```python
from build123d import *

# Parameters (mm, degrees)
SKETCH2_W           = 20
SKETCH2_H           = 20
SKETCH2_R           = 2.5
BOSS_EXTRUDE1_DEPTH = 250
SKETCH3_R           = 2.5
CUT_EXTRUDE1_DEPTH  = 251.99800796
SKETCH4_R           = 2.5
CUT_EXTRUDE2_DEPTH  = 251.99800796


with BuildPart() as part:
    # Sketch2 → Boss-Extrude1 (new body)
    with BuildSketch(Plane(origin=(0, 0, 0), x_dir=(1, 0, 0), z_dir=(0, 1, 0))):
        Rectangle(SKETCH2_W, SKETCH2_H)
        with Locations(Location((0, 0, 0), (0, 0, 270))):
            Circle(SKETCH2_R, mode=Mode.SUBTRACT)
    extrude(amount=BOSS_EXTRUDE1_DEPTH)

    # Sketch3 → Cut-Extrude1 (cut, through all)
    with BuildSketch(Plane.XY.offset(10)):
        with Locations((0, 5)):
            Circle(SKETCH3_R)
    extrude(amount=-CUT_EXTRUDE1_DEPTH, mode=Mode.SUBTRACT)

    # Sketch4 → Cut-Extrude2 (cut, through all)
    with BuildSketch(Plane.XY.offset(10)):
        with Locations((0, 75)):
            Circle(SKETCH4_R)
        with Locations((0, 85)):
            Circle(SKETCH4_R)
        with Locations((0, 150)):
            Circle(SKETCH4_R)
        with Locations((0, 160)):
            Circle(SKETCH4_R)
    extrude(amount=-CUT_EXTRUDE2_DEPTH, mode=Mode.SUBTRACT)


solid = part.part
```
Could you check a few things on this model? Use its own coordinates, in mm. Give positions to 0.01 mm unless a question says otherwise; leave off trailing zeros. Loops run counter-clockwise (first coordinate to the right, second up) from the corner with the lowest first, then second, coordinate; pieces in that order, holes last. Notation, with made-up numbers: (-2, -5.75) - (56, -5.75) arc R29 cw to (56, 14.25) - close; hole circle Ø1 at (-7.75, 74.25). An arc over 180 degrees is marked (long way). Use one line per item in the form item = value.
1. I'm going to push a flat-ended pin straight in: pin 1 Ø8 at (x, z) = (0, 0) entering from +Y. Where does the tip first touch, or does it pass through?
Response values:
pin_1 = 250
2. Thinking about a two-plate mould opening in Y: for faces 1 (the face through (2.11, 154.93, 1.34)), 2 (the face through (-2, 0, 2)), 3 (the face through (-2.5, 85.1, 6.2)), which applies, released by +Y, released by -Y, zero draft, split by the parting line, or undercut?
Response values:
face_1 = zero draft
face_2 = released by -Y
face_3 = undercut
3. I want a section at B-B (y = 109.5). Please give me the cut outline in (x, z), and give its area (3 significant figures).
Response values:
outline = (-10, -10) - (10, -10) - (10, 10) - (-10, 10) - close; hole circle Ø5 at (0, 0)
area = 380 mm²
4. I want a section at A-A (z = -4.75). Please give me the cut outline in (x, y), and give its area (3 significant figures).
Response values:
outline = (-10, 0) - (10, 0) - (10, 250) - (-10, 250) - close; hole circle Ø5 at (0, 5); hole circle Ø5 at (0, 75); hole circle Ø5 at (0, 85); hole circle Ø5 at (0, 150); hole circle Ø5 at (0, 160)
area = 4,900 mm²
5. I want a section at C-C (x = 0). Give the number of separate pieces and of enclosed holes in the cut face, and give its area (4 significant figures).
Response values:
separate_pieces = 12
enclosed_holes = 0
area = 3,375 mm²
6. I need wall thicknesses on probe 1 along Y at (x, z) = (0, 3.25); probe 2 along X at (y, z) = (150, 7.5); probe 3 along Y at (x, z) = (-1.75, -4.75). Which ranges of each line are inside material? Lowest first, please.
Response values:
probe_1 = 0 to 2.5, 7.5 to 72.5, 77.5 to 82.5, 87.5 to 147.5, 152.5 to 157.5, 162.5 to 250
probe_2 = -10 to -2.5, 2.5 to 10
probe_3 = 0 to 3.21, 6.79 to 73.21, 76.79 to 83.21, 86.79 to 148.21, 151.79 to 158.21, 161.79 to 250
